from build123d import *

# Parameters (mm, degrees)
BOSS_EXTRUDE1_DEPTH     = 11.5
SKETCH1_13_R            = 1.5
SKETCH1_13_R_2          = 1.25
BOSS_EXTRUDE2_DEPTH     = 7.75
BOSS_EXTRUDE3_DEPTH     = 7
SKETCH2_W               = 23
SKETCH2_H               = 23
BOSS_EXTRUDE4_DEPTH     = 120
SKETCH9_W               = 19.998553098
SKETCH9_H               = 11.329894336
CUT_EXTRUDE7_DEPTH      = 5
CUT_EXTRUDE7_DEPTH_BACK = 57
CUT_EXTRUDE8_START      = -8
SKETCH8_W               = 40.995866108
SKETCH8_H               = 19.999889565
SKETCH8_R               = 1.5
CUT_EXTRUDE8_DEPTH      = 20
SKETCH10_W              = 57.182789297
SKETCH10_H              = 20.379722455
CUT_EXTRUDE9_DEPTH      = 1
SKETCH11_W              = 59.739039785
SKETCH11_H              = 8
CUT_EXTRUDE10_DEPTH     = 40
SKETCH12_W              = 59.739039785
SKETCH12_H              = 8
CUT_EXTRUDE11_DEPTH     = 40
CUT_EXTRUDE12_DEPTH     = 57


with BuildPart() as part:
    # Sketch1 → Boss-Extrude1 (new body, symmetric)
    with BuildSketch(Plane(origin=(0, 0, 0), x_dir=(1, 0, 0), z_dir=(0, 1, 0))):
        with BuildLine():
            Line((6.824314586, 7.284360201), (6.824314586, 9.00020274))
            Line((6.824314586, 9.00020274), (-3.690467309, 9.00020274))
            Line((-3.690467309, 9.00020274), (-17.038497557, 11.5))
            Line((-17.038497557, 11.5), (-24.867971487, 11.5))
            Line((-24.867971487, 11.5), (-24.867971487, -11.5))
            Line((-24.867971487, -11.5), (-17.038497557, -11.5))
            Line((-17.038497557, -11.5), (-3.690467309, -9.00020274))
            Line((-3.690467309, -9.00020274), (6.824314586, -9.00020274))
            Line((6.824314586, -9.00020274), (6.824314586, -7.284360201))
            ThreePointArc((6.824314586, -7.284360201), (4.861171432, -6.879883717), (3.082035449, -5.956732906))
            Line((3.082035449, -5.956732906), (-3.422402494, -3.9))
            Line((-3.422402494, -3.9), (-19.513448301, -3.9))
            Line((-19.513448301, -3.9), (-19.513448301, 3.9))
            Line((-19.513448301, 3.9), (-3.422402494, 3.9))
            Line((-3.422402494, 3.9), (3.082035449, 5.956732906))
            ThreePointArc((3.082035449, 5.956732906), (4.861171432, 6.879883717), (6.824314586, 7.284360201))
        make_face()
    extrude(amount=BOSS_EXTRUDE1_DEPTH, both=True)

    # Sketch1_13 → Boss-Extrude2 (add, symmetric)
    with BuildSketch(Plane(origin=(0, 0, 0), x_dir=(1, 0, 0), z_dir=(0, 1, 0))):
        with BuildLine():
            Line((6.824314586, 3.971385595), (6.824314586, 7.284360201))
            ThreePointArc((6.824314586, 7.284360201), (4.861171432, 6.879883717), (3.082035449, 5.956732906))
            Line((3.082035449, 5.956732906), (-3.422402494, 3.9))
            Line((-3.422402494, 3.9), (-19.513448301, 3.9))
            Line((-19.513448301, 3.9), (-19.513448301, -3.9))
            Line((-19.513448301, -3.9), (-3.422402494, -3.9))
            Line((-3.422402494, -3.9), (3.082035449, -5.956732906))
            ThreePointArc((3.082035449, -5.956732906), (4.861171432, -6.879883717), (6.824314586, -7.284360201))
            Line((6.824314586, -7.284360201), (6.824314586, -3.971385595))
            ThreePointArc((6.824314586, -3.971385595), (3.301909035, 0), (6.824314586, 3.971385595))
        make_face()
        with Locations((-17.038497557, 0)):
            Circle(SKETCH1_13_R, mode=Mode.SUBTRACT)
        with Locations((-13.038497557, 0)):
            Circle(SKETCH1_13_R, mode=Mode.SUBTRACT)
        with Locations((-2.172402494, 0)):
            Circle(SKETCH1_13_R_2, mode=Mode.SUBTRACT)
    extrude(amount=BOSS_EXTRUDE2_DEPTH, both=True)

    # Sketch1_14 → Boss-Extrude3 (add, symmetric)
    with BuildSketch(Plane(origin=(0, 0, 0), x_dir=(1, 0, 0), z_dir=(0, 1, 0))):
        with BuildLine():
            Line((6.824314586, -3.971385595), (6.824314586, 3.971385595))
            ThreePointArc((6.824314586, 3.971385595), (3.301909035, 0), (6.824314586, -3.971385595))
        make_face()
    extrude(amount=BOSS_EXTRUDE3_DEPTH, both=True)

    # Sketch2 → Boss-Extrude4 (add)
    with BuildSketch(Plane.ZY.offset(24.867971487)):
        Rectangle(SKETCH2_W, SKETCH2_H)
    extrude(amount=BOSS_EXTRUDE4_DEPTH)

    # Sketch9 → Cut-Extrude7 (cut, two sides)
    with BuildSketch(Plane.ZY.offset(144.867971487)) as cut_extrude7_sk:
        with Locations((0.000723451, -5.664947168)):
            Rectangle(SKETCH9_W, SKETCH9_H)
    extrude(amount=CUT_EXTRUDE7_DEPTH, mode=Mode.SUBTRACT)
    extrude(cut_extrude7_sk.sketch, amount=-CUT_EXTRUDE7_DEPTH_BACK, mode=Mode.SUBTRACT)

    # Sketch8 → Cut-Extrude8 (cut)
    with BuildSketch(Plane.XZ.offset(11.5).offset(CUT_EXTRUDE8_START)):
        with Locations((-115.870038433, 5.5217e-05)):
            Rectangle(SKETCH8_W, SKETCH8_H)
        with Locations((-91.122105379, 5.125027608)):
            Circle(SKETCH8_R)
        with Locations((-91.121972212, -5.124917175)):
            Circle(SKETCH8_R)
        with Locations((-140.617971487, 5.125)):
            Circle(SKETCH8_R)
        with Locations((-140.617971487, -5.125)):
            Circle(SKETCH8_R)
    extrude(amount=-CUT_EXTRUDE8_DEPTH, mode=Mode.SUBTRACT)

    # Sketch10 → Cut-Extrude9 (cut)
    with BuildSketch(Plane.XZ.offset(11.5)):
        with Locations((-116.276576839, 0.092053876)):
            Rectangle(SKETCH10_W, SKETCH10_H)
    extrude(amount=-CUT_EXTRUDE9_DEPTH, mode=Mode.SUBTRACT)

    # Sketch11 → Cut-Extrude10 (cut)
    with BuildSketch(Plane(origin=(0, 11.5, 0), x_dir=(1, 0, 0), z_dir=(0, 1, 0))):
        with Locations((-52.611089146, 0)):
            Rectangle(SKETCH11_W, SKETCH11_H)
    extrude(amount=-CUT_EXTRUDE10_DEPTH, mode=Mode.SUBTRACT)

    # Sketch12 → Cut-Extrude11 (cut)
    with BuildSketch(Plane(origin=(0, 0, -11.5), x_dir=(-1, 0, 0), z_dir=(0, 0, -1))):
        with Locations((52.611089146, 0)):
            Rectangle(SKETCH12_W, SKETCH12_H)
    extrude(amount=-CUT_EXTRUDE11_DEPTH, mode=Mode.SUBTRACT)

    # Sketch9_12 → Cut-Extrude12 (cut)
    with BuildSketch(Plane.ZY.offset(144.867971487)):
        Polygon((10, 3.5), (11.5, 3.5), (11.5, 3.545517382), (11.5, 11.5), (10, 11.5), (-9.999842993, 11.5), (-11.5, 11.5), (-11.5, 3.5), (-10, 3.5), align=None)
    extrude(amount=-CUT_EXTRUDE12_DEPTH, mode=Mode.SUBTRACT)


solid = part.part
Geometry check sheet. Reference: the model listing, model coordinates, mm. A direction names the side the tool comes from. Coordinates: 2 decimals unless noted, no trailing zeros. Order: outer loops, then holes, each group sorted by start corner. A loop starts at its lowest first (then second) coordinate and runs counter-clockwise, first axis right, second up. Notation, with made-up numbers: (-16, 66) - (-12, 66) arc R27 cw to (-12, 88) - close; hole circle Ø7 at (3.5, -12). An arc over 180 degrees is marked (long way). One line per item, written item: value.
(1) Access from +Z, -Z, +X, -X, +Y, -Y to the whole of each face (thin tool, end or side, straight path). Record for faces 4 (the face through (-117, -4, 10)), 5 (the face through (-0.216, -9.599, -4.914)), 6 (the face through (2, 0, -9)), 7 (the face through (-11, 10, 3.9)).
Data:
face 4: -Y
face 5: +X, -Y
face 6: -Z, +X, +Y, -Y
face 7: +X, +Y
(2) Sectioned sample at B-B (y = 9.25). Enter the section's corners in (x, z), and give its area (3 significant figures).
Data:
outline: (-87.87, -11.5) - (-17.04, -11.5) - (-3.69, -9) - (6.82, -9) - (6.82, -7.28) arc R7.3 cw to (3.08, -5.96) - (-3.42, -3.9) - (-19.51, -3.9) - (-19.51, 3.9) - (-3.42, 3.9) - (3.08, 5.96) arc R7.3 cw to (6.82, 7.28) - (6.82, 9) - (-3.69, 9) - (-17.04, 11.5) - (-87.87, 11.5) - close; hole (-82.48, -4) - (-22.74, -4) - (-22.74, 4) - (-82.48, 4) - close
area: 1,370 mm^2
(3) Sectioned sample at D-D (z = 0). Count the separate pieces of the cut face and the enclosed holes in it, and give its area (3 significant figures).
Data:
separate pieces: 6
enclosed holes: 0
area: 525 mm^2
(4) Thickness scan on probe 1 along X at (y, z) = (-2.25, 0); probe 2 along X at (y, z) = (3, 5.25); probe 3 along Z at (x, y) = (-38.5, 5.5). Record the ranges inside material, lowest first. Write a range as from..to.
Data:
probe 1: x = -87.87..-82.48, -22.74..-18.54, -15.54..-14.54, -11.54..-3.42, -0.92..6.82
probe 2: x = -144.87..-142.11, -139.12..-136.37, -95.37..-92.62, -89.63..-82.48, -22.74..6.82
probe 3: z = -11.5..-4, 4..11.5
(5) Sectioned sample at C-C (x = -37.5). Enter the section's corners in (y, z), and give its area (3 significant figures).
Data:
outline: (-11.5, -11.5) - (-4, -11.5) - (-4, -4) - (-11.5, -4) - close; (-11.5, 4) - (-4, 4) - (-4, 11.5) - (-11.5, 11.5) - close; (4, -11.5) - (11.5, -11.5) - (11.5, -4) - (4, -4) - close; (4, 4) - (11.5, 4) - (11.5, 11.5) - (4, 11.5) - close
area: 225 mm^2
(6) Depth check by flat-ended pin: pin 1 Ø3 at (x, y) = (0.5, -5.5) entering from -Z; pin 2 Ø6 at (x, z) = (-93, 1.5) entering from -Y; pin 3 Ø1.1 at (y, z) = (9, -2) entering from +X. Enter the tip coordinate at first touch or a pass-through.
Data:
pin 1: stops at z = -9
pin 2: stops at y = 0
pin 3: stops at x = -19.51
(7) Release check for a two-part mould opening along Y. For faces 1 (the face through (-116.5, 3.5, 10.2)), 2 (the face through (-117, -6, -9.999)), 3 (the face through (-52, 4, 8)) record: +Y half, -Y half, draft (parallel to the pull), parting line (faces both ways), or undercut.
Data:
face 1: +Y half
face 2: draft
face 3: undercut
